```python
from build123d import *

# Parameters (mm, degrees)
SKETCH_1_R               = 7.5
EXTRUDE_1_DEPTH          = 16
SKETCH_2_R               = 10
SKETCH_2_R_2             = 7.5
EXTRUDE_2_DEPTH          = 4
SKETCH_3_R               = 17.5
SKETCH_3_R_2             = 10
CUT_EXTRUDE_1_DEPTH      = 3.5
SKETCH_4_R               = 17
CUT_EXTRUDE_2_DEPTH      = 3.5
FILLET_1_R               = 4
FILLET_2_R               = 2
FILLET_3_R               = 1
SKETCH_5_R               = 3.5
CUT_EXTRUDE_3_DEPTH      = 37
CUT_EXTRUDE_3_DEPTH_BACK = 8


with BuildPart() as part:
    # 草图1 → 凸台-拉伸1 (new body)
    with BuildSketch(Plane.XY):
        with BuildLine():
            Line((-40, 0), (-21, 0))
            Line((-21, 0), (-21, 15))
            ThreePointArc((-21, 15), (0, 36), (21, 15))
            Line((21, 15), (21, 0))
            Line((21, 0), (40, 0))
            Line((40, 0), (40, -7))
            Line((40, -7), (14.696938457, -7))
            Line((14.696938457, -7), (14.696938457, 0))
            ThreePointArc((14.696938457, 0), (0, -6), (-14.696938457, 0))
            Line((-14.696938457, 0), (-14.696938457, -7))
            Line((-14.696938457, -7), (-40, -7))
            Line((-40, -7), (-40, 0))
        make_face()
        with Locations((0, 15)):
            Circle(SKETCH_1_R, mode=Mode.SUBTRACT)
    extrude(amount=EXTRUDE_1_DEPTH)

    # 草图2 → 凸台-拉伸2 (add)
    with BuildSketch(Plane.XY.offset(16)):
        with Locations((0, 15)):
            Circle(SKETCH_2_R)
        with Locations((0, 15)):
            Circle(SKETCH_2_R_2, mode=Mode.SUBTRACT)
    extrude(amount=EXTRUDE_2_DEPTH)

    # 草图3 → 切除-拉伸1 (cut)
    with BuildSketch(Plane.XY.offset(16)):
        with Locations((0, 15)):
            Circle(SKETCH_3_R)
        with Locations((0, 15)):
            Circle(SKETCH_3_R_2, mode=Mode.SUBTRACT)
    extrude(amount=-CUT_EXTRUDE_1_DEPTH, mode=Mode.SUBTRACT)

    # 草图4 → 切除-拉伸2 (cut)
    with BuildSketch(Plane(origin=(0, 0, 0), x_dir=(-1, 0, 0), z_dir=(0, 0, -1))):
        with Locations((0, 15)):
            Circle(SKETCH_4_R)
    extrude(amount=-CUT_EXTRUDE_2_DEPTH, mode=Mode.SUBTRACT)

    # 圆角1
    fillet_1_edges = [part.edges().sort_by_distance(p)[0] for p in [
        (40, -3.5, 0),
        (-40, -3.5, 0),
        (40, -3.5, 16),
        (-40, -3.5, 16),
    ]]
    fillet(fillet_1_edges, radius=FILLET_1_R)

    # 圆角2
    fillet_2_edges = [part.edges().sort_by_distance(p)[0] for p in [
        (14.696938457, 0, 8),
        (-14.696938457, 0, 8),
    ]]
    fillet(fillet_2_edges, radius=FILLET_2_R)

    # 圆角3
    fillet_3_edges = [part.edges().sort_by_distance(p)[0] for p in [
        (-10, 15, 20),
        (-17.5, 15, 16),
        (-7.5, 15, 3.5),
        (17, 15, 0),
    ]]
    fillet(fillet_3_edges, radius=FILLET_3_R)

    # 草图5 → 切除-拉伸3 (cut, two sides)
    with BuildSketch(Plane(origin=(0, 0, 0), x_dir=(1, 0, 0), z_dir=(0, 1, 0))) as cut_extrude_3_sk:
        with Locations((-31.5, -8)):
            Circle(SKETCH_5_R)
        with Locations((31.5, -8)):
            Circle(SKETCH_5_R)
    extrude(amount=CUT_EXTRUDE_3_DEPTH, mode=Mode.SUBTRACT)
    extrude(cut_extrude_3_sk.sketch, amount=-CUT_EXTRUDE_3_DEPTH_BACK, mode=Mode.SUBTRACT)


solid = part.part
```
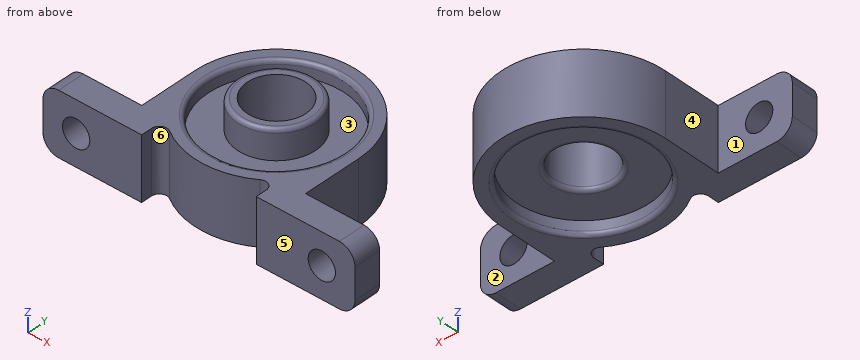
Source: CAD feature listing. Evaluate the final solid. Frame: model axes, mm. Face numbers are marked on the shaded views. A direction names the side the tool comes from. Give positions to 0.01 mm unless a question says otherwise; leave off trailing zeros. Loops run counter-clockwise (first coordinate to the right, second up) from the corner with the lowest first, then second, coordinate; pieces in that order, holes last. Notation, with made-up numbers: M -18,30 L 41,30 A23 cw 41,66 Z; hole C 76,-39 d7. An arc over 180 degrees is marked long. Put each result on its own line as item: value.
Q1. Reachability of the marked faces 1, 2 and 3 from +Z, -Z, +X, -X, +Y, -Y: full face, straight path, thin tool, end or side. Return the list, or none.
Response values:
face 1: +Z, -Z, -X, +Y
face 2: +Z, -Z, +X, +Y
face 3: +Z
Q2. Section C-C (z = 17.75). Return the cut outline in (x, y), and give its area (3 significant figures).
Response values:
outline: C 0,15 d20; hole C 0,15 d15
area: 137 mm²
Q3. Mould query, pull axis X, two halves, no side actions, for the marked faces 4, 5 and 6. Classes: released by +X, released by -X, zero draft, split by the parting line, or undercut.
Response values:
face 4: released by -X
face 5: zero draft
face 6: undercut
Q4. Section D-D (x = 0). Return the cut outline in (y, z).
Response values:
outline: M -6,0 L -3,0 A1 ccw -2,1 L -2,3.5 L 6.5,3.5 A1 ccw 7.5,4.5 L 7.5,20 L 6,20 A1 ccw 5,19 L 5,12.5 L -2.5,12.5 L -2.5,15 A1 ccw -3.5,16 L -6,16 Z; M 22.5,4.5 A1 ccw 23.5,3.5 L 32,3.5 L 32,1 A1 ccw 33,0 L 36,0 L 36,16 L 33.5,16 A1 ccw 32.5,15 L 32.5,12.5 L 25,12.5 L 25,19 A1 ccw 24,20 L 22.5,20 Z
Q5. Section A-A (z = 8). Return the cut outline in (x, y), and give its area (3 significant figures).
Response values:
outline: M -40,-7 L -35,-7 L -35,0 L -40,0 Z; M -28,-7 L -14.7,-7 L -14.7,-4.18 A2 cw -11.59,-2.51 A21 ccw 11.59,-2.51 A2 cw 14.7,-4.18 L 14.7,-7 L 28,-7 L 28,0 L 21,0 L 21,15 A21 ccw -21,15 L -21,0 L -28,0 Z; M 35,-7 L 40,-7 L 40,0 L 35,0 Z; hole C 0,15 d15
area: 1,530 mm²
Q6. Line query: probe 1 along Y at (x, z) = (0, 14.3); probe 2 along X at (y, z) = (-3, 6); probe 3 along Y at (x, z) = (0, 1.8). Output: solid intervals per line, ascending. Write a range as [from, to].
Response values:
probe 1: y = [-6, -2.5], [5, 7.5], [22.5, 25], [32.5, 36]
probe 2: x = [-40, -34.37], [-28.63, -14.31], [-10.82, 10.82], [14.31, 28.63], [34.37, 40]
probe 3: y = [-6, -2], [32, 36]
Q7. Pin query (flat end, axial travel): P1, Ø4, axis at x = -12, y = 21.5, coming from the -Z side; P2, Ø1.5, axis at y = 19.5, z = 16.5, coming from the -X side; P3, Ø4, axis at x = -12.5, z = 11.5, coming from the -Y side. Return the tip coordinate at first contact, or that it passes through.
Response values:
P1: stops at z = 3.5
P2: stops at x = -20.63
P3: stops at y = -3.31
Q8. Section B-B (x = 31.5). Return the cut outline in (y, z).
Response values:
outline: M -7,0 L 0,0 L 0,4.5 L -7,4.5 Z; M -7,11.5 L 0,11.5 L 0,16 L -7,16 Z
